Build history of the part. All positions in model axes, mm. Face numbers are marked on the shaded views. Give positions to 0.01 mm unless a question says otherwise; leave off trailing zeros. Loops run counter-clockwise (first coordinate to the right, second up) from the corner with the lowest first, then second, coordinate; pieces in that order, holes last.
1) Two-plate mould, pull along Z, no slides. Class the marked faces 1 and 2: +Z half, -Z half, draft (parallel to the pull), parting line (faces both ways), or undercut.
2) Flat gauge pins, fed straight in: P1, Ø4, axis at y = -4.5, z = -14.5, coming from the +X side; P2, Ø3, axis at x = 253.5, z = 3.5, coming from the -Y side; P3, Ø8, axis at x = 254, y = -10, coming from the -Z side; P4, Ø4, axis at x = 366.5, z = -7.5, coming from the +Y side. Where does each tip first touch, or does it go through?
3) Band-saw the part on C-C on z = 0. List the corners of the cut face in (x, y).
4) Band-saw the part on A-A on y = 0. List the corners of the cut face in (x, z).
5) Band-saw the part on B-B on x = 280.5. List the corners of the cut face in (y, z).
6) Wall check: line 1 (Y direction, x = 158, z = 0); line 2 (Z direction, x = 79, y = -13). Give the ranges that are in metal, low to high.
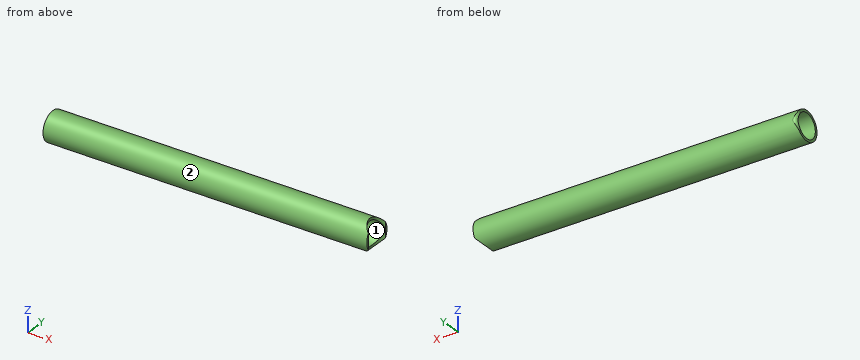
```python
from build123d import *

# Parameters (mm, degrees)
SKETCH1_R               = 21.082
SKETCH1_R_2             = 17.526
BOSS_EXTRUDE1_DEPTH     = 469.10625
CUT_EXTRUDE1_DEPTH      = 22.082
CUT_EXTRUDE1_DEPTH_BACK = 22.082
SKETCH3_R               = 21.082
CUT_EXTRUDE2_DEPTH      = 22.0820001
CUT_EXTRUDE2_DEPTH_BACK = 22.0820001


with BuildPart() as part:
    # Sketch1 → Boss-Extrude1 (new body)
    with BuildSketch(Plane(origin=(0, 0, 0), x_dir=(0, 0, -1), z_dir=(1, 0, 0))):
        Circle(SKETCH1_R)
        Circle(SKETCH1_R_2, mode=Mode.SUBTRACT)
    extrude(amount=BOSS_EXTRUDE1_DEPTH)

    # Sketch2 → Cut-Extrude1 (cut, two sides)
    with BuildSketch(Plane.XY) as cut_extrude1_sk:
        with BuildLine():
            Line((0, 21.082), (0, 14.732))
            ThreePointArc((0, 14.732), (1.859871939, 19.222128061), (6.35, 21.082))
            Line((6.35, 21.082), (0, 21.082))
        make_face()
    extrude(amount=CUT_EXTRUDE1_DEPTH, mode=Mode.SUBTRACT)
    extrude(cut_extrude1_sk.sketch, amount=-CUT_EXTRUDE1_DEPTH_BACK, mode=Mode.SUBTRACT)

    # Sketch3 → Cut-Extrude2 (cut, two sides)
    with BuildSketch(Plane.XY) as cut_extrude2_sk:
        with Locations((480.21875, 0)):
            Circle(SKETCH3_R)
    extrude(amount=CUT_EXTRUDE2_DEPTH, mode=Mode.SUBTRACT)
    extrude(cut_extrude2_sk.sketch, amount=-CUT_EXTRUDE2_DEPTH_BACK, mode=Mode.SUBTRACT)


solid = part.part
```
Findings below:
1. face 1: undercut
1. face 2: parting line
2. P1: passes through
2. P2: stops at y = -20.99
2. P3: stops at z = -20.21
2. P4: stops at y = 20.35
3. outline: (0, -21.08) - (469.11, -21.08) - (469.11, -17.92) arc R21.08 cw to (468.5, -17.53) - (0, -17.53) - close; (0.65, 17.53) - (468.5, 17.53) arc R21.08 cw to (469.11, 17.92) - (469.11, 21.08) - (6.35, 21.08) arc R6.35 ccw to start
4. outline: (0, -21.08) - (459.14, -21.08) - (459.14, -17.53) - (0, -17.53) - close; (0, 17.53) - (459.14, 17.53) - (459.14, 21.08) - (0, 21.08) - close
5. outline: circle Ø42.16 at (0, 0); hole circle Ø35.05 at (0, 0)
6. line 1: y = -21.08 to -17.53, 17.53 to 21.08
6. line 2: z = -16.6 to -11.75, 11.75 to 16.6
